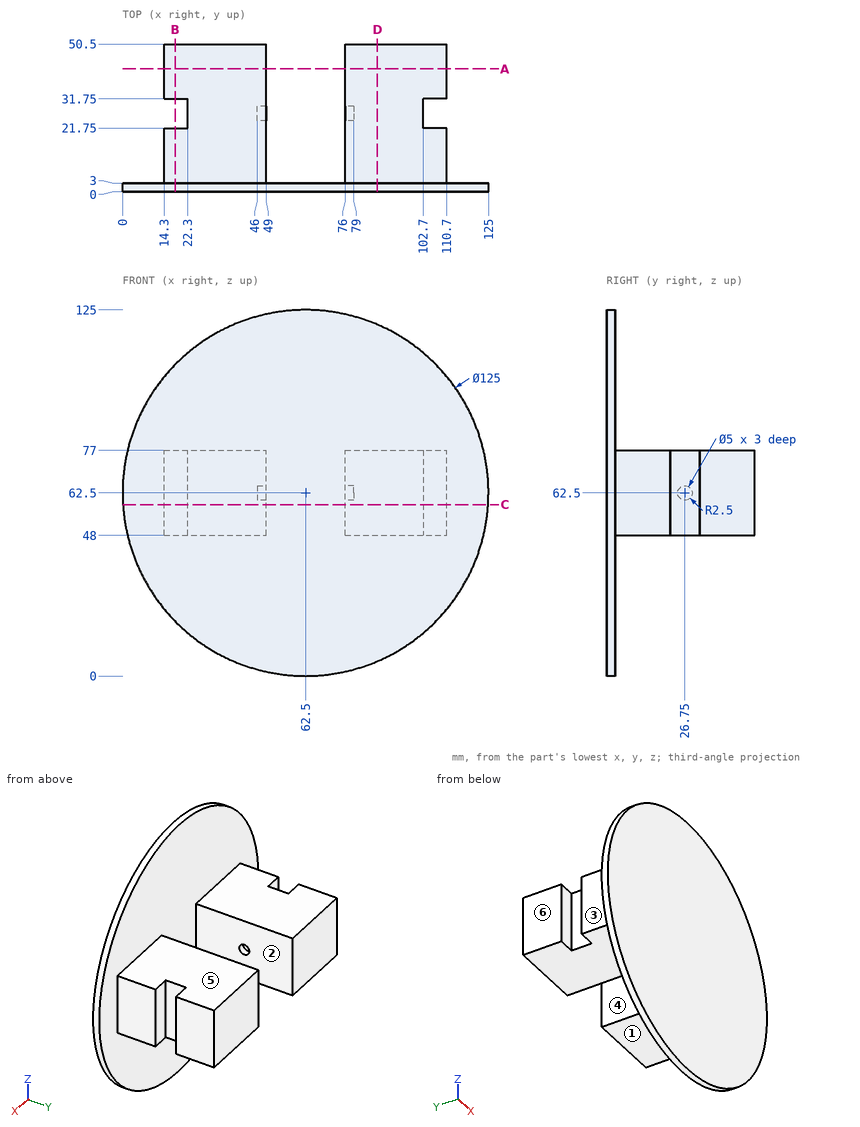
Verification items for this drawing (mm, ordinates from the low corner). A direction names the side the tool comes from. Give positions to 0.01 mm unless a question says otherwise; leave off trailing zeros. Loops run counter-clockwise (first coordinate to the right, second up) from the corner with the lowest first, then second, coordinate; pieces in that order, holes last. Notation, with made-up numbers: M 30.25,-14.5 L 84.25,-14.5 A11 cw 84.25,-7.5 Z; hole C 66.25,75.25 d4. An arc over 180 degrees is marked long. Answer as a JSON object with one key per item and string values. Group by question number.
Q1. Access from +Z, -Z, +X, -X, +Y, -Y to the whole of each face (thin tool, end or side, straight path). Record for the marked faces 4, 5 and 6.
Q2. Cross-section at C-C on z = 58.5. Record the cut outline in (x, y).
Q3. Cross-section at D-D on x = 87. Record the cut outline in (y, z), then the cut area to 3 significant figures.
Q4. Cross-section at B-B on x = 18. Record the cut outline in (y, z), then the cut area to 3 significant figures.
Q5. Go/stop test with flat-tipped pins: P1, Ø5, axis at x = 87, y = 40.5, coming from the +Z side; P2, Ø15, axis at y = 8.5, z = 59.5, coming from the +X side; P3, Ø20.5, axis at y = 12, z = 59, coming from the -X side; P4, Ø4, axis at x = 19, y = 28, coming from the +Z side. Record where each tip stops, or that it passes through.
Q6. Cross-section at A-A on y = 42. Record the cut outline in (x, z).
Q7. Material ranges on line 1 along Y through (x, z) = (48, 62.5); line 2 along Y through (x, z) = (110, 50); line 3 along Z through (x, y) = (47.15, 26.75), recorded low to high. Write a range as [from, to].
Q8. Release check for a two-part mould opening along X. For the marked faces 1, 2 and 3 record: released by +X, released by -X, zero draft, split by the parting line, or undercut.
Evaluation:
{
 "1": {"face 4": "+Z, -Z, +Y", "face 5": "+Z, +X, -X, +Y", "face 6": "+Z, -Z, -X, +Y"},
 "2": {"outline": "M 0.13,0 L 124.87,0 L 124.87,3 L 110.7,3 L 110.7,21.75 L 102.7,21.75 L 102.7,31.75 L 110.7,31.75 L 110.7,50.5 L 76,50.5 L 76,3 L 49,3 L 49,50.5 L 14.3,50.5 L 14.3,31.75 L 22.3,31.75 L 22.3,21.75 L 14.3,21.75 L 14.3,3 L 0.13,3 Z"},
 "3": {"outline": "M 0,5 L 3,5 L 3,48 L 50.5,48 L 50.5,77 L 3,77 L 3,120 L 0,120 Z", "area": "1,720 mm2"},
 "4": {"outline": "M 0,18.61 L 3,18.61 L 3,48 L 21.75,48 L 21.75,77 L 3,77 L 3,106.39 L 0,106.39 Z; M 31.75,48 L 50.5,48 L 50.5,77 L 31.75,77 Z", "area": "1,350 mm2"},
 "5": {"P1": "stops at z = 77", "P2": "stops at x = 125", "P3": "stops at x = 0", "P4": "passes through"},
 "6": {"outline": "M 14.3,48 L 49,48 L 49,77 L 14.3,77 Z; M 76,48 L 110.7,48 L 110.7,77 L 76,77 Z"},
 "7": {"line 1": "y = [0, 24.25], [29.25, 50.5]", "line 2": "y = [0, 21.75], [31.75, 50.5]", "line 3": "z = [48, 60], [65, 77]"},
 "8": {"face 1": "zero draft", "face 2": "undercut", "face 3": "released by -X"}
}
